Geometry: see drawing. Coordinates: mm, zero at the bounding-box minimum. A direction names the side the tool comes from. Give positions to 0.01 mm unless a question says otherwise; leave off trailing zeros. Write each loop counter-clockwise with the first axis right and the second up, starting at its lowest first coordinate (ties: lowest second). Pieces come first, ordered by that corner, then holes. Notation, with made-up numbers: (57.25, 73) - (94.25, 73) arc R16 ccw to (94.25, 97) - close; hole circle Ø7 at (62, 58). An arc over 180 degrees is marked (long way). One line per question, with ' | ' between items. Start each with the question number.
(1) Section D-D, the plane y = 4.35. Return loops of the section in (x, z).
(2) Section B-B, the plane z = 3.5. Return loops of the section in (x, y).
(3) Pin query (flat end, axial travel): pin 1 (3 mm diameter, centred on x = 6, z = 3.5, fed in from -Y); pin 2 (1.5 mm diameter, centred on y = 1.5, z = 2.5, fed in from +X); pin 3 (1.5 mm diameter, centred on x = 1, y = 0.5, fed in from -Z). Return the tip coordinate at first contact, or that it passes through.
(4) Access query for the marked faces 1 and 2. Directions: +Z, -Z, +X, -X, +Y, -Y. A direction counts if a zero-diameter tool reaches every point of the face in a straight line with its end or side. Return the directions, or none.
(5) Draft query along Y for the marked faces 3, 4, 5 and 6. Return one class per face: +Y half, -Y half, draft (parallel to the pull), parting line (faces both ways), or undercut.
(6) Ray query, line 1 (X direction, y = 1.5, z = 3.5); line 2 (X direction, y = 2.8, z = 3.5); line 3 (Y direction, x = 5.25, z = 0.5). Return the intervals inside material, ascending. Write a range as [from, to].
(7) Section A-A, the plane x = 3.5. Return loops of the section in (y, z).
(8) Section C-C, the plane y = 0.65. Return loops of the section in (x, z).
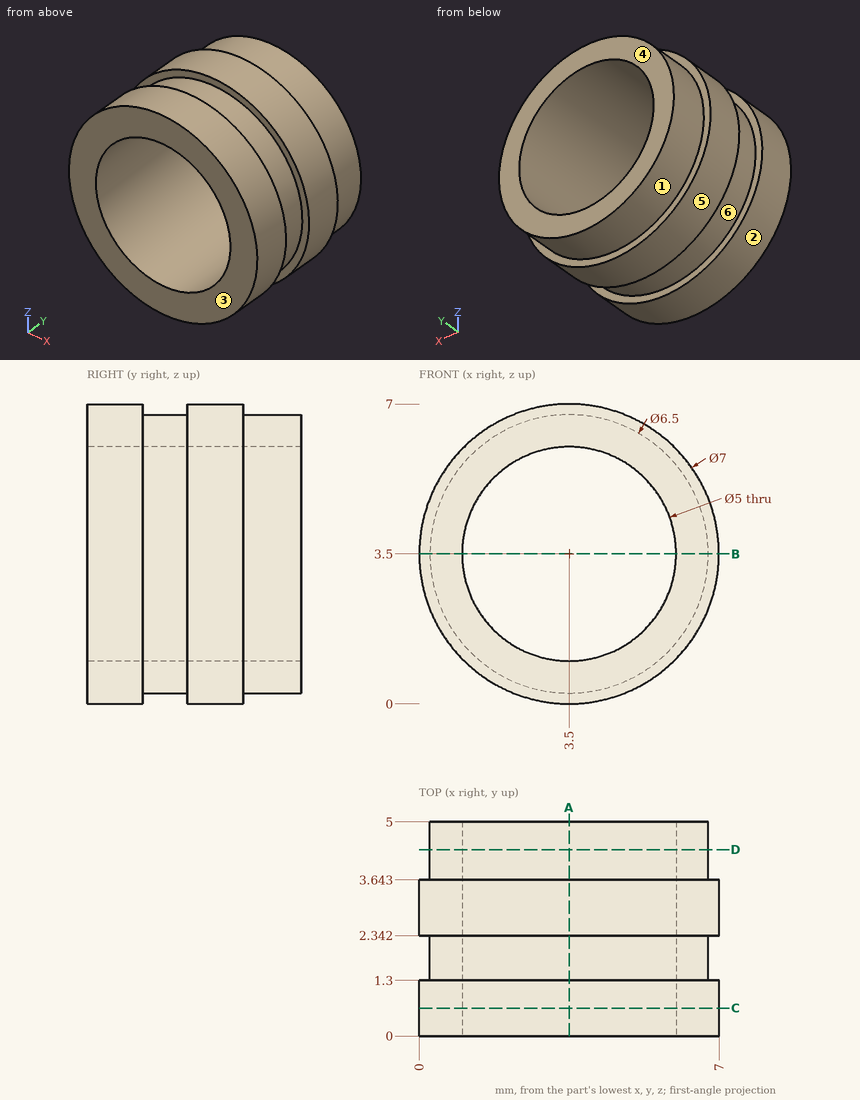
Check sheet entries:
1) outline: circle Ø6.5 at (3.5, 3.5); hole circle Ø5 at (3.5, 3.5)
2) outline: (0, 0) - (1, 0) - (1, 5) - (0.25, 5) - (0.25, 3.64) - (0, 3.64) - (0, 2.34) - (0.25, 2.34) - (0.25, 1.3) - (0, 1.3) - close; (6, 0) - (7, 0) - (7, 1.3) - (6.75, 1.3) - (6.75, 2.34) - (7, 2.34) - (7, 3.64) - (6.75, 3.64) - (6.75, 5) - (6, 5) - close
3) pin 1: y = 0 | pin 2: x = 6.99 | pin 3: z = 0.47
4) face 1: +Y | face 2: +Y, -Y
5) face 3: -Y half | face 4: +Y half | face 5: draft | face 6: undercut
6) line 1: [0.25, 1], [6, 6.75] | line 2: [0, 1], [6, 7] | line 3: [0, 1.3], [2.34, 3.64]
7) outline: (0, 0) - (1.3, 0) - (1.3, 0.25) - (2.34, 0.25) - (2.34, 0) - (3.64, 0) - (3.64, 0.25) - (5, 0.25) - (5, 1) - (0, 1) - close; (0, 6) - (5, 6) - (5, 6.75) - (3.64, 6.75) - (3.64, 7) - (2.34, 7) - (2.34, 6.75) - (1.3, 6.75) - (1.3, 7) - (0, 7) - close
8) outline: circle Ø7 at (3.5, 3.5); hole circle Ø5 at (3.5, 3.5)
